Work out the finished part from the listing and answer in its coordinate system (mm). A direction names the side the tool comes from. Round coordinates to 2 decimals unless told otherwise and drop trailing zeros. Answer in a Markdown table with one row per item.
```python
from build123d import *

# Parameters (mm, degrees)
SKETCH1_R           = 5.25
BOSS_EXTRUDE1_DEPTH = 8
FILLET1_SIZE        = 1.5
FILLET1_SIZE_2      = 3
FILLET2_R           = 5
CHAMFER1_SIZE2      = 0.798099646
CHAMFER1_SIZE       = 6.5
FILLET4_DEPTH       = 8
FILLET5_R           = 0.5
FILLET6_R           = 6
SKETCH2_R           = 1.85
CUT_EXTRUDE1_DEPTH  = 8
FILLET7_R           = 4


with BuildPart() as part:
    # Sketch1 → Boss-Extrude1 (new body)
    with BuildSketch(Plane(origin=(0, 0, 0), x_dir=(1, 0, 0), z_dir=(0, 1, 0))):
        Polygon((20, -7), (22, -5), (-4, 18), (-6, 18), (-6, 13), (-9, 10), (-9, 8.7), (-15.5, 8.7), (-15.5, 6.2), (-9, 1.7), (-9, -9), (2, -9), (10, -3), (16, -7), align=None)
        with Locations(Location((0, 0, 0), (0, 0, 270))):
            Circle(SKETCH1_R, mode=Mode.SUBTRACT)
    extrude(amount=BOSS_EXTRUDE1_DEPTH)

    # Fillet1
    # a fillet whose section is not a circle: 3, 1.5 mm, written as the material it takes off along each edge
    with BuildSketch(Plane(origin=(-6, -7.5, -18), x_dir=(1, 0, 0), z_dir=(0, 1, 0))) as fillet1_piece_1:
        with BuildLine():
            Bezier((FILLET1_SIZE, 0), (0, 0), (0, -FILLET1_SIZE_2), weights=[1, 0.707106781, 1])
            Line((0, -FILLET1_SIZE_2), (0, 0))
            Line((0, 0), (FILLET1_SIZE, 0))
        make_face()
    extrude(amount=23, mode=Mode.SUBTRACT)

    # Fillet2
    fillet2_edges = [part.edges().sort_by_distance(p)[0] for p in [
        (-6, 4, -13),
    ]]
    fillet(fillet2_edges, radius=FILLET2_R)

    # Chamfer1
    chamfer1_edges = [part.edges().sort_by_distance(p)[0] for p in [
        (-15.5, 4, -8.7),
    ]]
    chamfer1_side = [part.faces().sort_by_distance(p)[0] for p in [
        (-15.484038007, 4, -8.7),
    ]]
    chamfer(chamfer1_edges, length=CHAMFER1_SIZE - 0.0001, length2=CHAMFER1_SIZE2 - 0.0001, reference=chamfer1_side[0])  # a hair under: the kernel refuses the full size

    # Fillet4: read off the stored shape, not the designer's step
    # Fillet4 outline → Fillet4 (add)
    with BuildSketch(Plane(origin=(0, 0, 0), x_dir=(1, 0, 0), z_dir=(0, 1, 0))):
        with BuildLine():
            ThreePointArc((-11.153950106, 3.191196227), (-9.57110344, 1.40076867), (-9, -0.919764731))
            Line((-9, -0.919764731), (-9, 1.7))
            Line((-9, 1.7), (-11.153950106, 3.191196227))
        make_face()
        with BuildLine():
            Line((-9, 8.7), (-9, 10))
            ThreePointArc((-9, 10), (-10.428118078, 8.860869286), (-12.170105392, 8.310760001))
            Line((-12.170105392, 8.310760001), (-9, 8.7))
        make_face()
    extrude(amount=FILLET4_DEPTH)

    # Fillet5
    fillet5_edges = [part.edges().sort_by_distance(p)[0] for p in [
        (-15.5, 4, -6.2),
        (-15.5, 4, -7.902000354),
    ]]
    fillet(fillet5_edges, radius=FILLET5_R)

    # Fillet6
    fillet6_edges = [part.edges().sort_by_distance(p)[0] for p in [
        (10, 4, 3),
        (2, 4, 9),
        (-9, 4, 9),
    ]]
    fillet(fillet6_edges, radius=FILLET6_R)

    # Sketch2 → Cut-Extrude1 (cut)
    with BuildSketch(Plane(origin=(7.176763485, 0, -8.112863071), x_dir=(-0.7489965624903806, 0, -0.662573882203029), z_dir=(0.662573882203029, 0, -0.7489965624903806))):
        with Locations((7.92231613, 4)):
            Circle(SKETCH2_R)
        with Locations((-14.07768387, 4)):
            Circle(SKETCH2_R)
    extrude(amount=-CUT_EXTRUDE1_DEPTH, mode=Mode.SUBTRACT)

    # Fillet7
    fillet7_edges = [part.edges().sort_by_distance(p)[0] for p in [
        (20, 4, 7),
    ]]
    fillet(fillet7_edges, radius=FILLET7_R)


solid = part.part
```
1. Determine the mould class of faces 4 (the cylindrical face through (19.854, 4.056, 6.704)), 5 (the flat face through (3, 0, -5)), 6 (the cylindrical face through (-2.115, 5.56, -11.067)) for opening direction Y: released by +Y, released by -Y, zero draft, split by the parting line, or undercut.
Calculated:
| item | result |
|---|---|
| face 4 | zero draft |
| face 5 | released by -Y |
| face 6 | undercut |
2. The part is cut by section A-A (y = 3.5). Count the separate pieces of the cut face and the enclosed holes in it, plus the area to 4 significant figures.
Calculated:
| item | result |
|---|---|
| separate pieces | 2 |
| enclosed holes | 1 |
| area | 345.5 mm² |
3. A tool of negligible diameter and unlimited length cuts with its end or side. For faces 1 (the flat face through (5.08, 3.94, 6.69)), 2 (the flat face through (21.6, 3.9, 5.4)), 3 (the flat face through (-9, 4, 2)), from which of +Z, -Z, +X, -X, +Y, -Y can it reach the whole face along a straight path? Write none if from no direction.
Calculated:
| item | result |
|---|---|
| face 1 | +Z, +Y, -Y |
| face 2 | +Z, +X, +Y, -Y |
| face 3 | +Z, -X, +Y, -Y |
4. Given pin 1 (2 mm diameter, centred on x = 11, y = 6.5, fed in from +Z); pin 2 (0.6 mm diameter, centred on y = 3.5, z = 1.5, fed in from -X); pin 3 (2 mm diameter, centred on y = 7, z = -3.5, fed in from +X), each flat-ended and moving along its own axis, determine where each tip first touches the part or whether it passes through.
Calculated:
| item | result |
|---|---|
| pin 1 | stops at z = 4.62 |
| pin 2 | stops at x = -9 |
| pin 3 | stops at x = 13.52 |
5. Consider line 1 along X through (y, z) = (3, -9.75); line 2 along X through (y, z) = (5, 0); line 3 along X through (y, z) = (6.5, -6.5). Determine where each line is inside the solid, lowest interval first. Write a range as from..to.
Calculated:
| item | result |
|---|---|
| line 1 | x = -9.23..-4.03, 0.13..5.33 |
| line 2 | x = -9.09..-5.25, 5.25..16.35 |
| line 3 | x = -15.5..9 |
